Could you check a few things on this model? Use its own coordinates, in mm. A direction names the side the tool comes from. Coordinates: 2 decimals unless noted, no trailing zeros. Write each loop counter-clockwise with the first axis right and the second up, starting at its lowest first coordinate (ties: lowest second). Pieces come first, ordered by that corner, then holes.
```python
from build123d import *

# Parameters (mm, degrees)
BOSS_EXTRU_1_DEPTH      = 1.5
BOSS_EXTRU_2_DEPTH      = 6.35
ESQUISSE2_W             = 2.048679464
ESQUISSE2_H             = 2.722217918
ESQUISSE2_W_2           = 2.383965353
ESQUISSE2_H_2           = 1.994278708
BOSS_EXTRU_3_DEPTH      = 1.5
ESQUISSE3_R             = 1.3
ENL_V_MAT_EXTRU_1_DEPTH = 170.97185291


with BuildPart() as part:
    # Model → Boss.-Extru.1 (new body)
    with BuildSketch(Plane.XY):
        with BuildLine():
            Line((110.49, -34.813931), (110.49, -38.623931))
            Line((110.49, -38.623931), (110.49, -39.893931))
            Line((110.49, -39.893931), (110.49, -123.713931))
            add(Edge.make_bspline(
                [(109.746051, -125.509982), (110.222394, -125.03364), (110.49, -124.387581), (110.49, -123.713931)],
                knots=[0, 0, 0, 0, 1, 1, 1, 1], degree=3))
            add(Edge.make_bspline(
                [(107.95, -126.253931), (108.62365, -126.253931), (109.269709, -125.986325), (109.746051, -125.509982)],
                knots=[0, 0, 0, 0, 1, 1, 1, 1], degree=3))
            Line((107.95, -126.253931), (85.09, -126.253931))
            add(Edge.make_bspline(
                [(83.293949, -125.509982), (83.770291, -125.986325), (84.41635, -126.253931), (85.09, -126.253931)],
                knots=[0, 0, 0, 0, 1, 1, 1, 1], degree=3))
            add(Edge.make_bspline(
                [(82.55, -123.713931), (82.55, -124.387581), (82.817606, -125.03364), (83.293949, -125.509982)],
                knots=[0, 0, 0, 0, 1, 1, 1, 1], degree=3))
            Line((82.55, -123.713931), (82.55, -39.893931))
            Line((82.55, -39.893931), (82.55, -38.623931))
            Line((82.55, -38.623931), (82.55, -34.813931))
            add(Edge.make_bspline(
                [(82.921974, -33.915905), (82.683803, -34.154076), (82.55, -34.477106), (82.55, -34.813931)],
                knots=[0, 0, 0, 0, 1, 1, 1, 1], degree=3))
            add(Edge.make_bspline(
                [(83.82, -33.543931), (83.483175, -33.543931), (83.160146, -33.677734), (82.921974, -33.915905)],
                knots=[0, 0, 0, 0, 1, 1, 1, 1], degree=3))
            Line((83.82, -33.543931), (109.22, -33.543931))
            add(Edge.make_bspline(
                [(110.118026, -33.915905), (109.879854, -33.677734), (109.556825, -33.543931), (109.22, -33.543931)],
                knots=[0, 0, 0, 0, 1, 1, 1, 1], degree=3))
            add(Edge.make_bspline(
                [(110.49, -34.813931), (110.49, -34.477106), (110.356197, -34.154076), (110.118026, -33.915905)],
                knots=[0, 0, 0, 0, 1, 1, 1, 1], degree=3))
        make_face()
        with BuildLine():
            add(Edge.make_bspline(
                [(109.22, -36.083931), (109.22, -36.537658), (108.977939, -36.956919), (108.585, -37.183783)],
                knots=[0, 0, 0, 0, 1, 1, 1, 1], degree=3))
            add(Edge.make_bspline(
                [(108.585, -37.183783), (108.192061, -37.410647), (107.707939, -37.410647), (107.315, -37.183783)],
                knots=[0, 0, 0, 0, 1, 1, 1, 1], degree=3))
            add(Edge.make_bspline(
                [(107.315, -37.183783), (106.922061, -36.956919), (106.68, -36.537658), (106.68, -36.083931)],
                knots=[0, 0, 0, 0, 1, 1, 1, 1], degree=3))
            add(Edge.make_bspline(
                [(106.68, -36.083931), (106.68, -35.630204), (106.922061, -35.210942), (107.315, -34.984079)],
                knots=[0, 0, 0, 0, 1, 1, 1, 1], degree=3))
            add(Edge.make_bspline(
                [(107.315, -34.984079), (107.707939, -34.757215), (108.192061, -34.757215), (108.585, -34.984079)],
                knots=[0, 0, 0, 0, 1, 1, 1, 1], degree=3))
            add(Edge.make_bspline(
                [(108.585, -34.984079), (108.977939, -35.210942), (109.22, -35.630204), (109.22, -36.083931)],
                knots=[0, 0, 0, 0, 1, 1, 1, 1], degree=3))
        make_face(mode=Mode.SUBTRACT)
        with BuildLine():
            add(Edge.make_bspline(
                [(86.36, -36.083931), (86.36, -36.537658), (86.117939, -36.956919), (85.725, -37.183783)],
                knots=[0, 0, 0, 0, 1, 1, 1, 1], degree=3))
            add(Edge.make_bspline(
                [(85.725, -37.183783), (85.332061, -37.410647), (84.847939, -37.410647), (84.455, -37.183783)],
                knots=[0, 0, 0, 0, 1, 1, 1, 1], degree=3))
            add(Edge.make_bspline(
                [(84.455, -37.183783), (84.062061, -36.956919), (83.82, -36.537658), (83.82, -36.083931)],
                knots=[0, 0, 0, 0, 1, 1, 1, 1], degree=3))
            add(Edge.make_bspline(
                [(83.82, -36.083931), (83.82, -35.630204), (84.062061, -35.210942), (84.455, -34.984079)],
                knots=[0, 0, 0, 0, 1, 1, 1, 1], degree=3))
            add(Edge.make_bspline(
                [(84.455, -34.984079), (84.847939, -34.757215), (85.332061, -34.757215), (85.725, -34.984079)],
                knots=[0, 0, 0, 0, 1, 1, 1, 1], degree=3))
            add(Edge.make_bspline(
                [(85.725, -34.984079), (86.117939, -35.210942), (86.36, -35.630204), (86.36, -36.083931)],
                knots=[0, 0, 0, 0, 1, 1, 1, 1], degree=3))
        make_face(mode=Mode.SUBTRACT)
        with BuildLine():
            add(Edge.make_bspline(
                [(86.36, -123.713931), (86.36, -124.167658), (86.117939, -124.586919), (85.725, -124.813783)],
                knots=[0, 0, 0, 0, 1, 1, 1, 1], degree=3))
            add(Edge.make_bspline(
                [(85.725, -124.813783), (85.332061, -125.040647), (84.847939, -125.040647), (84.455, -124.813783)],
                knots=[0, 0, 0, 0, 1, 1, 1, 1], degree=3))
            add(Edge.make_bspline(
                [(84.455, -124.813783), (84.062061, -124.586919), (83.82, -124.167658), (83.82, -123.713931)],
                knots=[0, 0, 0, 0, 1, 1, 1, 1], degree=3))
            add(Edge.make_bspline(
                [(83.82, -123.713931), (83.82, -123.260204), (84.062061, -122.840942), (84.455, -122.614079)],
                knots=[0, 0, 0, 0, 1, 1, 1, 1], degree=3))
            add(Edge.make_bspline(
                [(84.455, -122.614079), (84.847939, -122.387215), (85.332061, -122.387215), (85.725, -122.614079)],
                knots=[0, 0, 0, 0, 1, 1, 1, 1], degree=3))
            add(Edge.make_bspline(
                [(85.725, -122.614079), (86.117939, -122.840942), (86.36, -123.260204), (86.36, -123.713931)],
                knots=[0, 0, 0, 0, 1, 1, 1, 1], degree=3))
        make_face(mode=Mode.SUBTRACT)
        with BuildLine():
            add(Edge.make_bspline(
                [(109.22, -123.713931), (109.22, -124.167658), (108.977939, -124.586919), (108.585, -124.813783)],
                knots=[0, 0, 0, 0, 1, 1, 1, 1], degree=3))
            add(Edge.make_bspline(
                [(108.585, -124.813783), (108.192061, -125.040647), (107.707939, -125.040647), (107.315, -124.813783)],
                knots=[0, 0, 0, 0, 1, 1, 1, 1], degree=3))
            add(Edge.make_bspline(
                [(107.315, -124.813783), (106.922061, -124.586919), (106.68, -124.167658), (106.68, -123.713931)],
                knots=[0, 0, 0, 0, 1, 1, 1, 1], degree=3))
            add(Edge.make_bspline(
                [(106.68, -123.713931), (106.68, -123.260204), (106.922061, -122.840942), (107.315, -122.614079)],
                knots=[0, 0, 0, 0, 1, 1, 1, 1], degree=3))
            add(Edge.make_bspline(
                [(107.315, -122.614079), (107.707939, -122.387215), (108.192061, -122.387215), (108.585, -122.614079)],
                knots=[0, 0, 0, 0, 1, 1, 1, 1], degree=3))
            add(Edge.make_bspline(
                [(108.585, -122.614079), (108.977939, -122.840942), (109.22, -123.260204), (109.22, -123.713931)],
                knots=[0, 0, 0, 0, 1, 1, 1, 1], degree=3))
        make_face(mode=Mode.SUBTRACT)
    extrude(amount=BOSS_EXTRU_1_DEPTH)

    # Esquisse1 → Boss.-Extru.2 (add)
    with BuildSketch(Plane(origin=(0, 0, 0), x_dir=(-1, 0, 0), z_dir=(0, 0, -1))):
        with BuildLine():
            Line((-110.49, -31.152890146), (-82.55, -31.152890146))
            ThreePointArc((-82.55, -31.152890146), (-81.135786438, -31.738676584), (-80.55, -33.152890146))
            Line((-80.55, -33.152890146), (-80.55, -125.263931))
            ThreePointArc((-80.55, -125.263931), (-81.135786438, -126.678144562), (-82.55, -127.263931))
            Line((-82.55, -127.263931), (-110.49, -127.263931))
            ThreePointArc((-110.49, -127.263931), (-111.904213562, -126.678144562), (-112.49, -125.263931))
            Line((-112.49, -125.263931), (-112.49, -33.152890146))
            ThreePointArc((-112.49, -33.152890146), (-111.904213562, -31.738676584), (-110.49, -31.152890146))
        make_face()
        with BuildLine():
            Line((-109.49, -33.543931), (-83.55, -33.543931))
            ThreePointArc((-83.55, -33.543931), (-82.842893219, -33.836824219), (-82.55, -34.543931))
            Line((-82.55, -34.543931), (-82.55, -124.253931))
            ThreePointArc((-82.55, -124.253931), (-83.135786438, -125.668144562), (-84.55, -126.253931))
            Line((-84.55, -126.253931), (-108.49, -126.253931))
            ThreePointArc((-108.49, -126.253931), (-109.904213562, -125.668144562), (-110.49, -124.253931))
            Line((-110.49, -124.253931), (-110.49, -34.543931))
            ThreePointArc((-110.49, -34.543931), (-110.197106781, -33.836824219), (-109.49, -33.543931))
        make_face(mode=Mode.SUBTRACT)
    extrude(amount=-BOSS_EXTRU_2_DEPTH)

    # Esquisse2 → Boss.-Extru.3 (add)
    with BuildSketch(Plane.XY.offset(1.5)):
        Polygon((82.862908546, -122.803540967), (81.718920114, -124.049976123), (82.862908546, -126.448936938), (85.492374492, -126.781888794), (85.441151129, -125.817182132), (83.793466299, -125.023220012), (83.059264769, -123.828008219), align=None)
        with Locations((82.84166356, -34.077464167)):
            Rectangle(ESQUISSE2_W, ESQUISSE2_H)
        with Locations((109.83167143, -33.789106507)):
            Rectangle(ESQUISSE2_W_2, ESQUISSE2_H_2)
        Polygon((111.079756548, -122.69864172), (110.01722417, -123.503842038), (109.201933768, -125.195788786), (107.319834078, -125.55652456), (107.178740755, -126.670800036), (110.27455623, -126.615412866), (111.506281277, -125.468783374), align=None)
    extrude(amount=-BOSS_EXTRU_3_DEPTH)

    # Esquisse3 → Enlèv. mat.-Extru.1 (cut, through all)
    with BuildSketch(Plane(origin=(0, 0, 0), x_dir=(-1, 0, 0), z_dir=(0, 0, -1))):
        with Locations((-107.952359108, -36.080520753)):
            Circle(ESQUISSE3_R)
        with Locations((-85.119999339, -36.08524195)):
            Circle(ESQUISSE3_R)
        with Locations((-107.979999813, -123.71323395)):
            Circle(ESQUISSE3_R)
        with Locations((-85.119999826, -123.713259066)):
            Circle(ESQUISSE3_R)
    extrude(amount=-ENL_V_MAT_EXTRU_1_DEPTH, mode=Mode.SUBTRACT)


solid = part.part
```
1. I want a section at C-C on x = 93.5. Please give me the cut outline in (y, z).
Verdict:
outline: (-127.26, 0) - (-31.15, 0) - (-31.15, 6.35) - (-33.54, 6.35) - (-33.54, 1.5) - (-126.25, 1.5) - (-126.25, 6.35) - (-127.26, 6.35) - close
2. For pin 1 (8 mm diameter, centred on x = 97.5, y = -75.5, fed in from +Z); pin 2 (2 mm diameter, centred on x = 85.12, y = -36.09, fed in from -Z), each with a flat end and sliding along its axis, tell me the tip position at first contact or that it passes through.
Verdict:
pin 1: stops at z = 1.5
pin 2: passes through
3. I want a section at B-B on y = -74.5. Please give me the cut outline in (x, z).
Verdict:
outline: (80.55, 0) - (112.49, 0) - (112.49, 6.35) - (110.49, 6.35) - (110.49, 1.5) - (82.55, 1.5) - (82.55, 6.35) - (80.55, 6.35) - close
4. I want a section at A-A on z = 3.75. Please give me the cut outline in (x, y), plus the area to 3 significant figures.
Verdict:
outline: (80.55, -125.26) arc R2 ccw to (82.55, -127.26) - (110.49, -127.26) arc R2 ccw to (112.49, -125.26) - (112.49, -33.15) arc R2 ccw to (110.49, -31.15) - (82.55, -31.15) arc R2 ccw to (80.55, -33.15) - close; hole (82.55, -124.25) arc R2 ccw to (84.55, -126.25) - (108.49, -126.25) arc R2 ccw to (110.49, -124.25) - (110.49, -34.54) arc R1 ccw to (109.49, -33.54) - (83.55, -33.54) arc R1 ccw to (82.55, -34.54) - close
area: 478 mm2
5. Please list where these lines run through material, in increasing order: line 1 along Y through (x, z) = (85.12, 0.45); line 2 along X through (y, z) = (-65, 6); line 3 along Y through (x, z) = (89, 2.75).
Verdict:
line 1: y = -127.26 to -125.01, -122.41 to -37.39, -34.79 to -31.15
line 2: x = 80.55 to 82.55, 110.49 to 112.49
line 3: y = -127.26 to -126.25, -33.54 to -31.15
6. On a 3-axis mill with a long thin cutter (end or side, diameter ignored), from which of +Z, -Z, +X, -X, +Y, -Y can I reach the whole of each face in a straight line? I mean faces 1 (the face through (97, -79, 1.5)), 2 (the face through (97, -31.153, 3)). Say none if no direction works.
Verdict:
face 1: +Z
face 2: +Z, -Z, +X, -X, +Y
7. If we mould it in two halves opening along X, with no side actions, what happens to faces 3 (the face through (112.49, -80, 3)), 4 (the face through (97, -33.544, 4)), 5 (the face through (81.151, -31.723, 3.131)), 6 (the face through (83.12, -125.65, 3.89))? For each: pulls with the +X half, pulls with the -X half, needs draft (parallel to the pull), parting line crosses it, or undercut.
Verdict:
face 3: pulls with the +X half
face 4: undercut
face 5: pulls with the -X half
face 6: undercut
